Model file for the job. Use its own axes, mm. Give positions to 0.01 mm unless a question says otherwise; leave off trailing zeros. Order: outer loops, then holes, each group sorted by start corner. A loop starts at its lowest first (then second) coordinate and runs counter-clockwise, first axis right, second up. Notation, with made-up numbers: (71.25, 67) - (108.25, 67) arc R30 cw to (108.25, 97) - close; hole circle Ø7 at (87, 33.25). An arc over 180 degrees is marked (long way). Use CSV: the item, a comma, the result in double quotes. Start each with the question number.
(1) Band-saw the part on B-B, the plane z = 0. Count the separate pieces of the cut face and the enclosed holes in it, then the cut area to 3 significant figures.
(2) Drop a flat-ended pin along its axis: pin 1 Ø5.5 at (x, z) = (-76.2, 0) entering from -Y. Give the stop position or say it passes through.
(3) Band-saw the part on A-A, the plane x = 76.2. Give the cut face in (y, z), then the cut area to 3 significant figures.
(4) Probe L1, parallel to Z at x = 76.2, y = 1.2; L2, parallel to Z at x = 3.5, y = 3.9; L3, parallel to X at y = 4.8, z = 7. List the from-to ranges inside material, lowest first.
from build123d import *

# Parameters (mm, degrees)
SKETCH1_W           = 177.8
SKETCH1_H           = 25.4
BOSS_EXTRUDE1_DEPTH = 6
CUT_EXTRUDE2_DEPTH  = 91.002777735
FILLET1_R           = 6.35
SKETCH5_R           = 4.6355
CUT_EXTRUDE3_DEPTH  = 91.002777735


with BuildPart() as part:
    # Sketch1 → Boss-Extrude1 (new body)
    with BuildSketch(Plane(origin=(0, 0, 0), x_dir=(1, 0, 0), z_dir=(0, 1, 0))):
        Rectangle(SKETCH1_W, SKETCH1_H)
    extrude(amount=BOSS_EXTRUDE1_DEPTH)

    # Sketch4 → Cut-Extrude2 (cut, through all)
    with BuildSketch(Plane.XZ):
        with BuildLine():
            Line((-53.975, 3.175), (-47.625, 3.175))
            ThreePointArc((-47.625, 3.175), (-44.45, 0), (-47.625, -3.175))
            Line((-47.625, -3.175), (-53.975, -3.175))
            ThreePointArc((-53.975, -3.175), (-57.15, 0), (-53.975, 3.175))
        make_face()
        with BuildLine():
            Line((-28.575, 3.175), (-22.225, 3.175))
            ThreePointArc((-22.225, 3.175), (-19.05, 0), (-22.225, -3.175))
            Line((-22.225, -3.175), (-28.575, -3.175))
            ThreePointArc((-28.575, -3.175), (-31.75, 0), (-28.575, 3.175))
        make_face()
        with BuildLine():
            Line((-3.175, 3.175), (3.175, 3.175))
            ThreePointArc((3.175, 3.175), (6.35, 0), (3.175, -3.175))
            Line((3.175, -3.175), (-3.175, -3.175))
            ThreePointArc((-3.175, -3.175), (-6.35, 0), (-3.175, 3.175))
        make_face()
        with BuildLine():
            Line((22.225, 3.175), (28.575, 3.175))
            ThreePointArc((28.575, 3.175), (31.75, 0), (28.575, -3.175))
            Line((28.575, -3.175), (22.225, -3.175))
            ThreePointArc((22.225, -3.175), (19.05, 0), (22.225, 3.175))
        make_face()
        with BuildLine():
            Line((47.625, 3.175), (53.975, 3.175))
            ThreePointArc((53.975, 3.175), (57.15, 0), (53.975, -3.175))
            Line((53.975, -3.175), (47.625, -3.175))
            ThreePointArc((47.625, -3.175), (44.45, 0), (47.625, 3.175))
        make_face()
    extrude(amount=-CUT_EXTRUDE2_DEPTH, mode=Mode.SUBTRACT)

    # Fillet1
    fillet1_edges = [part.edges().sort_by_distance(p)[0] for p in [
        (-88.9, 3, -12.7),
        (88.9, 3, -12.7),
        (88.9, 3, 12.7),
        (-88.9, 3, 12.7),
    ]]
    fillet(fillet1_edges, radius=FILLET1_R)

    # Sketch5 → Cut-Extrude3 (cut, through all)
    with BuildSketch(Plane(origin=(0, 6, 0), x_dir=(1, 0, 0), z_dir=(0, 1, 0))):
        with Locations(Location((-76.2, 0, 0), (0, 0, 270))):
            Circle(SKETCH5_R)
    cut_extrude3 = extrude(amount=-CUT_EXTRUDE3_DEPTH, mode=Mode.SUBTRACT)

    # Mirror1: Cut-Extrude3 across plane
    add(cut_extrude3.mirror(Plane(origin=(0, 0, 0), x_dir=(0, 0, 1), z_dir=(1, 0, 0))), mode=Mode.SUBTRACT)


solid = part.part
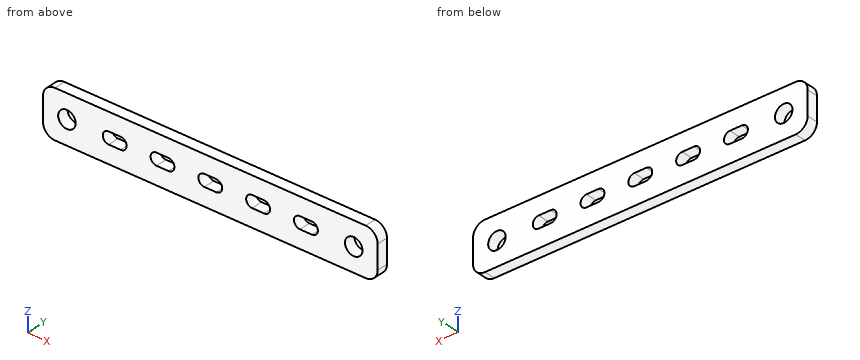
Answer block:
1,separate pieces,"8"
1,enclosed holes,"0"
1,area,"575 mm2"
2,pin 1,"passes through"
3,outline,"(0, -12.7) - (6, -12.7) - (6, -4.64) - (0, -4.64) - close; (0, 4.64) - (6, 4.64) - (6, 12.7) - (0, 12.7) - close"
3,area,"96.8 mm2"
4,L1,"z = -12.7 to -4.64, 4.64 to 12.7"
4,L2,"z = -12.7 to -3.16, 3.16 to 12.7"
4,L3,"x = -88.87 to 88.87"
